Part model, mm, in its own coordinate system. Face numbers are marked on the shaded views. A direction names the side the tool comes from. Give positions to 0.01 mm unless a question says otherwise; leave off trailing zeros. Write each loop counter-clockwise with the first axis right and the second up, starting at its lowest first coordinate (ties: lowest second). Pieces come first, ordered by that corner, then holes. Notation, with made-up numbers: M 25.5,72 L 36.5,72 A32 cw 36.5,100 Z; hole C -34.75,7 d8. An arc over 180 degrees is marked long. Use CSV: the item, a comma, the result in double quotes. Start each with the question number.
1. Band-saw the part on B-B, the plane x = 0. List the corners of the cut face in (y, z).
2. Band-saw the part on A-A, the plane z = 0. List the corners of the cut face in (x, y).
3. Band-saw the part on C-C, the plane y = 8.5. List the corners of the cut face in (x, z), then the cut area to 3 significant figures.
4. Band-saw the part on D-D, the plane x = 17. List the corners of the cut face in (y, z).
5. Drill centre lines: line 1 along Z through (x, y) = (0, 7); line 2 along Y through (x, z) = (-8.5, 2.5); line 3 along Y through (x, z) = (-7.5, 8.5). Where is each one in solid material? Low to high. Write a range as from..to.
6. 3-axis set-ups, long thin cutter, end or side, ignore diameter. For the marked faces 1 and 2: which of +Z, -Z, +X, -X, +Y, -Y reach the whole face in a straight line?
7. Drop flat-ended pins along their axis: pin 1 Ø2 at (y, z) = (3.5, 15.5) entering from +X; pin 2 Ø1 at (y, z) = (2, -5) entering from +X; pin 3 Ø1.7 at (y, z) = (9, 0) entering from +X; pin 4 Ø2.5 at (x, z) = (-17, 0) entering from -Y. Give the stop position or say it passes through.
Solid Edge part; units mm, degrees
sketch "Sketch1" plane through (0, 0, 0) normal (0, -1, 0) x (1, 0, 0)
  circle A0 centre (0, 0) radius 21.5
extrude "Protrusion1" add sketch "Sketch1" against normal blind 4
hole "Hole_1" at (-17, 4, 0) direction (0, -1, 0) diameter 3 end through all
hole "Hole1" at (17, 4, 0) direction (0, -1, 0) diameter 3 end through all
sketch "Sketch2" plane through (0, 4, 0) normal (0, 1, 0) x (0, 0, -1)
  circle A0 centre (0, 0) radius 10
extrude "ExtrudedProtrusion_2" add sketch "Sketch2" along normal blind 6
sketch "Sketch3" plane through (0, 10, 0) normal (0, 1, 0) x (-1, 0, 0)
  circle A0 centre (0, 0) radius 4
extrude "ExtrudedProtrusion_3" add sketch "Sketch3" along normal blind 7
sketch "Sketch4" plane through (0, 17, 0) normal (0, 1, 0) x (0, 0, -1)
  line L0 (-1.092, 1.1) -> (1.092, 1.1)
  arc A0 (1.092, 1.1) -> (-1.092, 1.1) centre (0, 0) cw
extrude "ExtrudedCutout_1" cut sketch "Sketch4" against normal blind 11
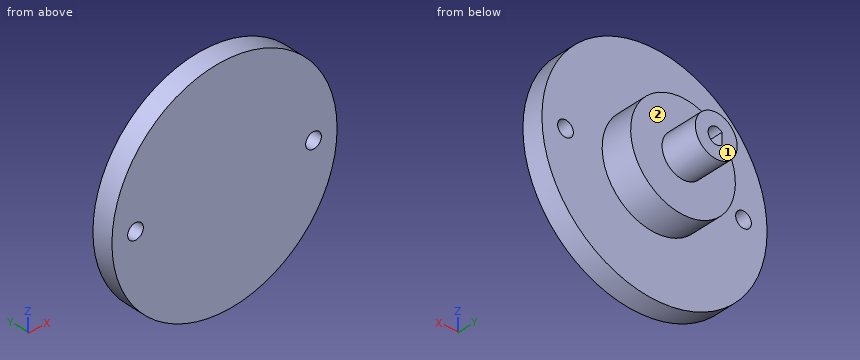
Output:
1,outline,"M 0,-21.5 L 4,-21.5 L 4,-10 L 10,-10 L 10,-4 L 17,-4 L 17,-1.55 L 6,-1.55 L 6,1.55 L 17,1.55 L 17,4 L 10,4 L 10,10 L 4,10 L 4,21.5 L 0,21.5 Z"
2,outline,"M -21.5,0 L -18.5,0 L -18.5,4 L -21.5,4 Z; M -15.5,0 L 15.5,0 L 15.5,4 L 10,4 L 10,10 L 4,10 L 4,17 L 1.55,17 L 1.55,6 L -1.1,6 L -1.1,17 L -4,17 L -4,10 L -10,10 L -10,4 L -15.5,4 Z; M 18.5,0 L 21.5,0 L 21.5,4 L 18.5,4 Z"
3,outline,"C 0,0 d20; hole M -1.1,-1.09 A1.55 ccw long -1.1,1.09 Z"
3,area,"307 mm²"
4,outline,"M 0,-13.16 L 4,-13.16 L 4,-1.5 L 0,-1.5 Z; M 0,1.5 L 4,1.5 L 4,13.16 L 0,13.16 Z"
5,line 1,"z = -10..-1.55, 1.55..10"
5,line 2,"y = 0..10"
5,line 3,"y = 0..4"
6,face 1,"+Z, -Z, +X, -X, +Y"
6,face 2,"+Y"
7,pin 1,"stops at x = 15.87"
7,pin 2,"stops at x = 21.02"
7,pin 3,"stops at x = 10"
7,pin 4,"passes through"
